from build123d import *

# Parameters (mm, degrees)
F0_W     = 50.8
F0_H     = 31.75
F1_DEPTH = 31.75
F2_W     = 19.05
F2_H     = 19.05
F3_DEPTH = 19.05
F4_DEPTH = 19.05
F6_DEPTH = 12.7
F8_DEPTH = 12.7


with BuildPart() as f1:
    # F0 (on Front) → F1 (new body)
    with BuildSketch(Plane.XZ):
        with Locations((25.4, 15.875)):
            Rectangle(F0_W, F0_H)
    extrude(amount=F1_DEPTH)

    # F2 (on face) → F3 (cut)
    with BuildSketch(Plane.XZ.offset(31.75)):
        with Locations((41.275, 22.225)):
            Rectangle(F2_W, F2_H)
    extrude(amount=-F3_DEPTH, mode=Mode.SUBTRACT)

    # F2 (on face) → F4 (cut)
    with BuildSketch(Plane.XZ.offset(31.75)):
        with Locations((9.525, 22.225)):
            Rectangle(F2_W, F2_H)
    extrude(amount=-F4_DEPTH, mode=Mode.SUBTRACT)

    # F5 (on face) → F6 (cut)
    with BuildSketch(Plane.YZ.offset(31.75)):
        Polygon((-31.75, 12.7), (-12.7, 31.75), (-31.75, 31.75), align=None)
    extrude(amount=-F6_DEPTH, mode=Mode.SUBTRACT)

    # F7 (on face) → F8 (cut)
    with BuildSketch(Plane.XZ.offset(12.7)):
        Polygon((50.8, 31.75), (31.75, 31.75), (50.8, 12.7), align=None)
    extrude(amount=-F8_DEPTH, mode=Mode.SUBTRACT)


solid = f1.part
The listing builds one solid part. Answer for the finished solid, in the listing's coordinates (mm). A direction names the side the tool comes from. Coordinates: 2 decimals unless noted, no trailing zeros. Order: outer loops, then holes, each group sorted by start corner. A loop starts at its lowest first (then second) coordinate and runs counter-clockwise, first axis right, second up.
Q1. A cutting plane is placed at C-C, the plane x = 11. Write down the section's boundary in (y, z), and give its area (3 significant figures).
Q2. Given P1, Ø5.5, axis at x = 37, z = 23.5, coming from the -Y side; P2, Ø2, axis at x = 8.5, y = -24.5, coming from the +Z side; P3, Ø5, axis at x = 29, y = -20.5, coming from the +Z side, each flat-ended and moving along its own axis, determine where each tip first touches the part or whether it passes through.
Q3. A cutting plane is placed at A-A, the plane y = -19.5. Write down the section's boundary in (x, z).
Q4. A cutting plane is placed at D-D, the plane x = 22.5. Write down the section's boundary in (y, z).
Q5. Consider line 1 (Z direction, x = 39, y = -17.5); line 2 (X direction, y = -27, z = 13.5); line 3 (Y direction, x = 43, z = 15). Determine where each line is inside the solid, lowest interval first.
Q6. A cutting plane is placed at B-B, the plane z = 16.5. Write down the section's boundary in (x, y), and give its area (3 significant figures).
Q7. Which of the six approach directions +Z, -Z, +X, -X, +Y, -Y give full straight-line access (tool end or side, diameter ignored) to faces 1 (the face through (37, -12.7, 18)), 2 (the face through (41.1, -6.4, 22.4)), 3 (the face through (9, -22, 12.7))?
Answers follow:
1. outline: (-31.75, 0) - (0, 0) - (0, 31.75) - (-12.7, 31.75) - (-12.7, 12.7) - (-31.75, 12.7) - close
1. area: 645 mm2
2. P1: stops at y = -12.7
2. P2: stops at z = 12.7
2. P3: stops at z = 26.45
3. outline: (0, 0) - (50.8, 0) - (50.8, 12.7) - (31.75, 12.7) - (31.75, 24.95) - (19.05, 24.95) - (19.05, 12.7) - (0, 12.7) - close
4. outline: (-31.75, 0) - (0, 0) - (0, 31.75) - (-12.7, 31.75) - (-31.75, 12.7) - close
5. line 1: z = 0 to 12.7
5. line 2: x = 19.05 to 31.75
5. line 3: y = -12.7 to 0
6. outline: (0, -12.7) - (19.05, -12.7) - (19.05, -27.95) - (31.75, -27.95) - (31.75, -12.7) - (47, -12.7) - (47, 0) - (0, 0) - close
6. area: 791 mm2
7. face 1: +Z, +X, -Y
7. face 2: +Z, +X, +Y, -Y
7. face 3: +Z, -X, -Y
